```python
from build123d import *

# Parameters (mm, degrees)
F1_W     = 58.76257
F1_H     = 51.44095
F1_W_2   = 38.76257
F1_H_2   = 31.44095
F2_DEPTH = 25
F0_W     = 58.76257
F0_H     = 51.44095
F0_W_2   = 38.76257
F0_H_2   = 31.44095
F3_DEPTH = 2


with BuildPart() as f2:
    # F1 (on face) → F2 (new body)
    with BuildSketch(Plane.XZ):
        Rectangle(F1_W, F1_H)
        Rectangle(F1_W_2, F1_H_2, mode=Mode.SUBTRACT)
    extrude(amount=F2_DEPTH)

    # F0 (on Front) + F1 (on face) → F3 (join)
    with BuildSketch(Plane.XZ):
        Rectangle(F0_W, F0_H)
        Rectangle(F0_W_2, F0_H_2, mode=Mode.SUBTRACT)
    with BuildSketch(Plane.XZ):
        Rectangle(F1_W_2, F1_H_2)
    extrude(amount=F3_DEPTH)


solid = f2.part
```
The listing builds one solid part. Answer for the finished solid, in the listing's coordinates (mm). A direction names the side the tool comes from. Coordinates: 2 decimals unless noted, no trailing zeros. Loops run counter-clockwise (first coordinate to the right, second up) from the corner with the lowest first, then second, coordinate; pieces in that order, holes last. Notation, with made-up numbers: M -16,82 L 2,82 A21 cw 2,92 Z; hole C -2,75 d7. An arc over 180 degrees is marked long. Answer as CSV lines item,"result". Start each with the question number.
(1) Given pin 1 (9.5 mm diameter, centred on x = -5, z = -3, fed in from -Y), flat-ended and moving along its own axis, determine where the tip first touches the part or whether it passes through.
(2) The part is cut by section B-B (z = -14). Give the vertices of the cut face in (x, y).
(3) For faces 1 (the flat face through (19.381, -13, 0)), 2 (the flat face through (0, 0, 0)), determine the directions among +Z, -Z, +X, -X, +Y, -Y from which every point of the face is accessible in a straight line to the end or side of a thin tool.
(4) The mould has two halves that part along Z. Classify faces 3 (the flat face through (29.381, -12, 0)), 4 (the flat face through (0, -2, 0)), 5 (the flat face through (0, -12, -25.72)): pulls with the +Z half, pulls with the -Z half, needs draft (parallel to the pull), parting line crosses it, or undercut.
(5) The part is cut by section A-A (y = -15.25). Give the vertices of the cut face in (x, z).
(6) Find the intervals of material crossed by L1, parallel to X at y = -9.25, z = 10.5; L2, parallel to Z at x = 12, y = -4.5; L3, parallel to Y at x = -16, z = 3, in increasing order. Write a range as [from, to].
(7) The part is cut by section C-C (x = 3). Give the vertices of the cut face in (y, z).
Determined:
1,pin 1,"y = -2"
2,outline,"M -29.38,-25 L -19.38,-25 L -19.38,-2 L 19.38,-2 L 19.38,-25 L 29.38,-25 L 29.38,0 L -29.38,0 Z"
3,face 1,"-Y"
3,face 2,"+Z, -Z, +X, -X, +Y"
4,face 3,"needs draft"
4,face 4,"undercut"
4,face 5,"pulls with the -Z half"
5,outline,"M -29.38,-25.72 L 29.38,-25.72 L 29.38,25.72 L -29.38,25.72 Z; hole M -19.38,-15.72 L 19.38,-15.72 L 19.38,15.72 L -19.38,15.72 Z"
6,L1,"[-29.38, -19.38], [19.38, 29.38]"
6,L2,"[-25.72, -15.72], [15.72, 25.72]"
6,L3,"[-2, 0]"
7,outline,"M -25,-25.72 L 0,-25.72 L 0,25.72 L -25,25.72 L -25,15.72 L -2,15.72 L -2,-15.72 L -25,-15.72 Z"
